Geometry check sheet. Reference: the model listing, model coordinates, mm. Give positions to 0.01 mm unless a question says otherwise; leave off trailing zeros. Write each loop counter-clockwise with the first axis right and the second up, starting at its lowest first coordinate (ties: lowest second). Pieces come first, ordered by that corner, then holes. Notation, with made-up numbers: (83, 51.5) - (103, 51.5) arc R31 cw to (103, 85.5) - close; hole circle Ø1 at (42.25, -6.5). An arc over 180 degrees is marked (long way). Write item = value, one per line. Start each with the question number.
(1) Thickness scan on L1, parallel to X at y = -9.5, z = 535; L2, parallel to X at y = -16, z = 192. Record the ranges inside material, lowest first.
(2) Section check A-A, the plane z = 76. Enter the section's corners in (x, y).
(3) Section check B-B, the plane x = 1.5. Enter the section's corners in (y, z), plus the area to 3 significant figures.
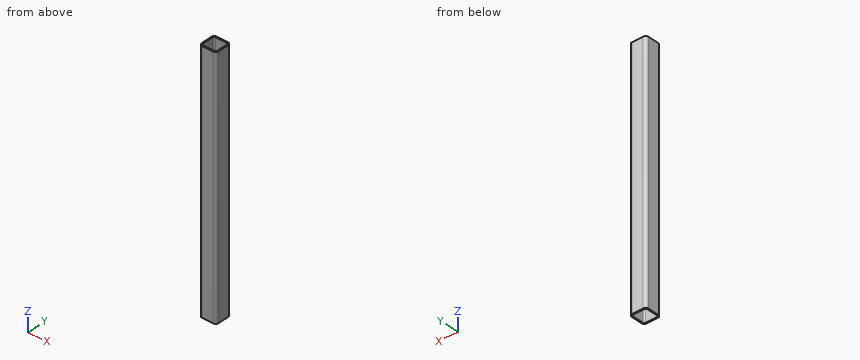
Autodesk Inventor part; units mm, degrees
ref_plane "Start plane" through (0, 0, 30) normal (0, 0, 1) x (1, 0, 0)
ref_plane "End plane" through (0, 0, 621) normal (0, 0, 1) x (1, 0, 0)
ref_plane "Work Plane5" through (29.2, 615, 621) normal (0, 0, 1) x (1, 0, 0)
ref_plane "Start plane" through (0, 0, 30) normal (0, 0, 1) x (1, 0, 0)
ref_plane "End plane" through (0, 0, 621) normal (0, 0, 1) x (1, 0, 0)
sketch "Sketch" plane through (0, 0, 0) normal (0, 0, 1) x (1, 0, 0)
  line L0 (-20, -13.4) -> (-20, 13.4)
  line L1 (-13.4, 20) -> (13.4, 20)
  line L2 (20, 13.4) -> (20, -13.4)
  line L3 (13.4, -20) -> (-13.4, -20)
  arc A0 (-20, -13.4) -> (-13.4, -20) centre (-13.4, -13.4) ccw
  arc A1 (-13.4, 20) -> (-20, 13.4) centre (-13.4, 13.4) ccw
  arc A2 (20, 13.4) -> (13.4, 20) centre (13.4, 13.4) ccw
  arc A3 (13.4, -20) -> (20, -13.4) centre (13.4, -13.4) ccw
  arc A4 (-13.4, 17) -> (-17, 13.4) centre (-13.4, 13.4) ccw
  line L4 (-13.4, 17) -> (13.4, 17)
  arc A5 (17, 13.4) -> (13.4, 17) centre (13.4, 13.4) ccw
  line L5 (17, 13.4) -> (17, -13.4)
  arc A6 (13.4, -17) -> (17, -13.4) centre (13.4, -13.4) ccw
  line L6 (13.4, -17) -> (-13.4, -17)
  arc A7 (-17, -13.4) -> (-13.4, -17) centre (-13.4, -13.4) ccw
  line L7 (-17, -13.4) -> (-17, 13.4)
  line L8 (0, 22.0873) -> (0, -22.0873) construction
  line L9 (-22.0873, 0) -> (22.0873, 0) construction
  dimension "d7" = 6.6
  dimension "d10" = 40
  dimension "d11" = 40
  dimension "d12" = 3
  dimension "d15" = 20
  dimension "d16" = 20
extrude "Body" add sketch "Sketch" along normal up to surface (591 mm away) from surface at 30
sketch "Sketch3" plane through (0, 0, 0) normal (0, 0, 1) x (1, 0, 0)
  line L0 (0, 0) -> (10, 0)
ref_plane "Work Plane3" through (0, 0, 0) normal (0, -1, 0) x (1, 0, 0)
sketch "Sketch4" plane through (0, 0, 0) normal (0, -1, 0) x (1, 0, 0)
  line L0 (-2, 30) -> (12, 30)
  line L1 (-2, 621) -> (12, 621)
  dimension "d18" = 591
ref_plane "Work Plane5" through (29.2, 615, 621) normal (0, 0, 1) x (1, 0, 0)
split "Split2" plane through (29.2, 615, 621) removes the side toward (0, 0, 1)
ref_plane "Work Plane6" through (29.2, -235, 30) normal (0, 0, -1) x (-1, 0, 0)
split "Split3" plane through (29.2, -235, 30) removes the side toward (0, 0, -1)
equation "\"d7\" = G_IR"
equation "\"d10\" = G_H"
equation "\"d11\" = G_W"
equation "\"d12\" = G_T"
equation "\"d15\" = 0.5 * d10"
equation "\"d16\" = 0.5 * d11"
equation "\"d3\" = G_L"
equation "\"G_W\" = 40"
equation "\"G_H\" = 40"
equation "\"G_T\" = 3"
equation "\"G_IR\" = 6.6"
equation "\"G_L\" = d18"
equation "\"d14\" = G_OFFSET_END + B_L"
equation "\"B_L\" = 651"
properties part number "DIN EN 10305-5 - 40 x 40 x 3  - 591" material "Steel, Mild"
Model answer:
q1.L1 = -20 to -17, 17 to 20
q1.L2 = -19.47 to -15.89, 15.89 to 19.47
q2.outline = (-20, -13.4) arc R6.6 ccw to (-13.4, -20) - (13.4, -20) arc R6.6 ccw to (20, -13.4) - (20, 13.4) arc R6.6 ccw to (13.4, 20) - (-13.4, 20) arc R6.6 ccw to (-20, 13.4) - close; hole (-17, -13.4) arc R3.6 ccw to (-13.4, -17) - (13.4, -17) arc R3.6 ccw to (17, -13.4) - (17, 13.4) arc R3.6 ccw to (13.4, 17) - (-13.4, 17) arc R3.6 ccw to (-17, 13.4) - close
q3.outline = (-20, 30) - (-17, 30) - (-17, 621) - (-20, 621) - close; (17, 30) - (20, 30) - (20, 621) - (17, 621) - close
q3.area = 3,550 mm²
